For this review, take the finished solid that the model builds, in its own axes (mm). Coordinates: 2 decimals unless noted, no trailing zeros. Loops run counter-clockwise (first coordinate to the right, second up) from the corner with the lowest first, then second, coordinate; pieces in that order, holes last. Notation, with made-up numbers: (-38, -30.75) -> (2, -30.75) arc R6 ccw to (2, -24.75) -> close; hole circle Ø7 at (-13.75, 45.5). An arc over 180 degrees is marked (long way). Use a Markdown table: item, result.
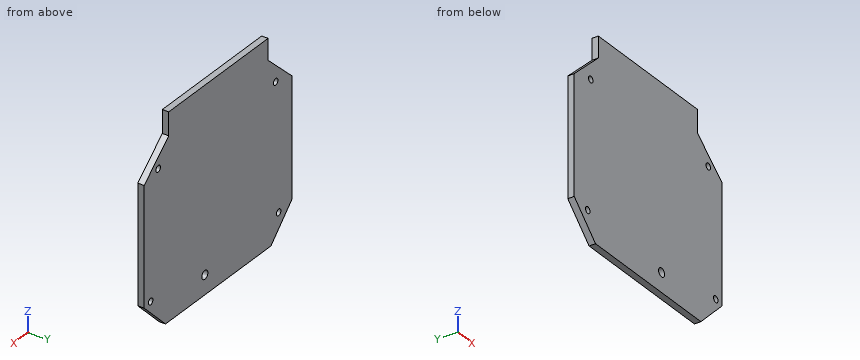
from build123d import *

# Parameters (mm, degrees)
SKETCH_1_R      = 1.5
SKETCH_1_R_2    = 2
EXTRUDE_1_DEPTH = 3


with BuildPart() as part:
    # 草图1 → 凸台-拉伸1 (new body)
    with BuildSketch(Plane(origin=(0, 0, 0), x_dir=(1, 0, 0), z_dir=(0, 1, 0))):
        Polygon((14.14, 0), (84.14, 0), (98.28, -14.14), (98.28, -69.14), (82, -83.28), (82, -94), (16, -94), (16, -84.14), (0, -69.14), (0, -14.14), align=None)
        with Locations(Location((9, -12.5, 0), (0, 0, 270))):
            Circle(SKETCH_1_R, mode=Mode.SUBTRACT)
        with Locations(Location((94, -15, 0), (0, 0, 270))):
            Circle(SKETCH_1_R, mode=Mode.SUBTRACT)
        with Locations(Location((11, -72, 0), (0, 0, 270))):
            Circle(SKETCH_1_R, mode=Mode.SUBTRACT)
        with Locations(Location((89, -72, 0), (0, 0, 270))):
            Circle(SKETCH_1_R, mode=Mode.SUBTRACT)
        with Locations(Location((58, -9, 0), (0, 0, 270))):
            Circle(SKETCH_1_R_2, mode=Mode.SUBTRACT)
    extrude(amount=EXTRUDE_1_DEPTH)


solid = part.part
(1) Take a section at A-A on z = 9. Write out the cut boundary in (x, y).
Found:
| item | result |
|---|---|
| outline | (5.14, 0) -> (56, 0) -> (56, 3) -> (5.14, 3) -> close; (60, 0) -> (93.14, 0) -> (93.14, 3) -> (60, 3) -> close |
(2) For line 1 along X through (y, z) = (0.7, 12.5); line 2 along X through (y, z) = (1.85, 15); line 3 along Z through (x, y) = (83.5, 0.6), list the stretches that pass through material, from the lowest coordinate up.
Found:
| item | result |
|---|---|
| line 1 | x = 1.64 to 7.5, 10.5 to 96.64 |
| line 2 | x = 0 to 92.5, 95.5 to 98.28 |
| line 3 | z = 0 to 81.98 |
(3) Take a section at D-D on z = 72. Write out the cut boundary in (x, y), plus the area to 3 significant figures.
Found:
| item | result |
|---|---|
| outline | (3.05, 0) -> (9.5, 0) -> (9.5, 3) -> (3.05, 3) -> close; (12.5, 0) -> (87.5, 0) -> (87.5, 3) -> (12.5, 3) -> close; (90.5, 0) -> (94.99, 0) -> (94.99, 3) -> (90.5, 3) -> close |
| area | 258 mm^2 |
(4) Take a section at C-C on y = 2.1. Write out the cut boundary in (x, z).
Found:
| item | result |
|---|---|
| outline | (0, 14.14) -> (14.14, 0) -> (84.14, 0) -> (98.28, 14.14) -> (98.28, 69.14) -> (82, 83.28) -> (82, 94) -> (16, 94) -> (16, 84.14) -> (0, 69.14) -> close; hole circle Ø3 at (9, 12.5); hole circle Ø3 at (11, 72); hole circle Ø4 at (58, 9); hole circle Ø3 at (89, 72); hole circle Ø3 at (94, 15) |
(5) Take a section at B-B on x = 58. Write out the cut boundary in (y, z).
Found:
| item | result |
|---|---|
| outline | (0, 0) -> (3, 0) -> (3, 7) -> (0, 7) -> close; (0, 11) -> (3, 11) -> (3, 94) -> (0, 94) -> close |
